The listing builds one solid part. Answer for the finished solid, in the listing's coordinates (mm). Round coordinates to 2 decimals unless told otherwise and drop trailing zeros. Write each loop counter-clockwise with the first axis right and the second up, starting at its lowest first coordinate (ties: lowest second). Pieces come first, ordered by that corner, then holes. Notation, with made-up numbers: (25, 21) - (30, 21) arc R19 cw to (30, 42) - close; hole circle Ø11 at (-22, 12.5). An arc over 180 degrees is marked (long way). Return JSON: item names as keys, results as strings. Group by question number.
(1) Each of these flat-tipped pins is pushed along its axis until it touches: pin 1 (0.7 mm diameter, centred on x = 4, z = -1.5, fed in from +Y); pin 2 (0.5 mm diameter, centred on x = 11.5, z = -2, fed in from +Y). Where does it stop, or does it pass through?
(2) Find the intervals of material crossed by line 1 along Z through (x, y) = (8.75, 3); line 2 along Y through (x, z) = (21.5, -1.6); line 3 along Y through (x, z) = (12, -1.85), in increasing order. Write a range as [from, to].
(3) Section A-A, the plane x = 11.5 is taken. Write down the section's boundary in (y, z).
(4) Section B-B, the plane y = 7 is taken. Give the number of separate pieces and of enclosed holes in the cut face, then the cut area to 3 significant figures.
```python
from build123d import *

# Parameters (mm, degrees)
SKETCH1_W                  = 25.4
SKETCH1_H                  = 3.556
BOSS_EXTRUDE1_DEPTH        = 8.636
SKETCH2_W                  = 0.635
SKETCH2_H                  = 0.635
CUT_EXTRUDE1_DEPTH         = 6.35
CHAMFER1_SIZE              = 0.508
LPATTERN1_COUNT            = 10
LPATTERN1_PITCH            = 2.54
CHAMFER1_OF_LPATTERN1_SIZE = 0.508


with BuildPart() as part:
    # Sketch1 → Boss-Extrude1 (new body)
    with BuildSketch(Plane(origin=(0, 0, 0), x_dir=(1, 0, 0), z_dir=(0, 1, 0))):
        with Locations((12.7, 1.778)):
            Rectangle(SKETCH1_W, SKETCH1_H)
    extrude(amount=BOSS_EXTRUDE1_DEPTH)

    # Sketch2 → Cut-Extrude1 (cut)
    with BuildSketch(Plane(origin=(0, 8.636, 0), x_dir=(1, 0, 0), z_dir=(0, 1, 0))):
        with Locations((1.27, 1.778)):
            Rectangle(SKETCH2_W, SKETCH2_H)
    cut_extrude1 = extrude(amount=-CUT_EXTRUDE1_DEPTH, mode=Mode.SUBTRACT)

    # Chamfer1
    chamfer1_edges = [part.edges().sort_by_distance(p)[0] for p in [
        (1.5875, 8.636, -1.778),
        (1.27, 8.636, -2.0955),
        (0.9525, 8.636, -1.778),
        (1.27, 8.636, -1.4605),
    ]]
    chamfer(chamfer1_edges, length=CHAMFER1_SIZE)

    # LPattern1: Cut-Extrude1 ×10
    with Locations(*[(i * LPATTERN1_PITCH, 0, 0) for i in range(1, LPATTERN1_COUNT)]):
        add(cut_extrude1, mode=Mode.SUBTRACT)

    # Chamfer1 of LPattern1
    chamfer1_of_lpattern1_edges = [part.edges().sort_by_distance(p)[0] for p in [
        (4.1275, 8.636, -1.778),
        (3.81, 8.636, -2.0955),
        (3.4925, 8.636, -1.778),
        (3.81, 8.636, -1.4605),
        (6.6675, 8.636, -1.778),
        (6.35, 8.636, -2.0955),
        (6.0325, 8.636, -1.778),
        (6.35, 8.636, -1.4605),
        (9.2075, 8.636, -1.778),
        (8.89, 8.636, -2.0955),
        (8.5725, 8.636, -1.778),
        (8.89, 8.636, -1.4605),
        (11.7475, 8.636, -1.778),
        (11.43, 8.636, -2.0955),
        (11.1125, 8.636, -1.778),
        (11.43, 8.636, -1.4605),
        (14.2875, 8.636, -1.778),
        (13.97, 8.636, -2.0955),
        (13.6525, 8.636, -1.778),
        (13.97, 8.636, -1.4605),
        (16.8275, 8.636, -1.778),
        (16.51, 8.636, -2.0955),
        (16.1925, 8.636, -1.778),
        (16.51, 8.636, -1.4605),
        (19.3675, 8.636, -1.778),
        (19.05, 8.636, -2.0955),
        (18.7325, 8.636, -1.778),
        (19.05, 8.636, -1.4605),
        (21.9075, 8.636, -1.778),
        (21.59, 8.636, -2.0955),
        (21.2725, 8.636, -1.778),
        (21.59, 8.636, -1.4605),
        (24.4475, 8.636, -1.778),
        (24.13, 8.636, -2.0955),
        (23.8125, 8.636, -1.778),
        (24.13, 8.636, -1.4605),
    ]]
    chamfer(chamfer1_of_lpattern1_edges, length=CHAMFER1_OF_LPATTERN1_SIZE)


solid = part.part
```
Working result:
{
 "1": {"pin 1": "stops at y = 8.44", "pin 2": "stops at y = 8.28"},
 "2": {"line 1": "z = [-3.56, -2.1], [-1.46, 0]", "line 2": "y = [0, 2.29]", "line 3": "y = [0, 8.38]"},
 "3": {"outline": "(0, -3.56) - (8.64, -3.56) - (8.64, -2.6) - (8.13, -2.1) - (2.29, -2.1) - (2.29, -1.46) - (8.13, -1.46) - (8.64, -0.95) - (8.64, 0) - (0, 0) - close"},
 "4": {"separate pieces": "1", "enclosed holes": "10", "area": "86.3 mm^2"}
}
